Source: CAD feature listing. Evaluate the final solid. Frame: model axes, mm. Face numbers are marked on the shaded views. A direction names the side the tool comes from. Round coordinates to 2 decimals unless told otherwise and drop trailing zeros. Loops run counter-clockwise (first coordinate to the right, second up) from the corner with the lowest first, then second, coordinate; pieces in that order, holes last. Notation, with made-up numbers: M 78.5,13.5 L 126.5,13.5 A20 cw 126.5,42.5 Z; hole C 72,73.25 d5. An arc over 180 degrees is marked long. Write each question's results on one line, items separated by ' | '. Start each with the question number.
1. Set-up query: the marked faces 4, 5 and 6. Return all of +Z, -Z, +X, -X, +Y, -Y with unobstructed straight access to the full face (end or side cutting, diameter ignored); none if empty.
2. Section A-A on x = 2. Output: boundary loops of the cut face in (y, z).
3. Contact query for flat-ended pins moving along their axis: pin 1 Ø10 at (x, z) = (-55, 33) entering from -Y; pin 2 Ø10 at (x, y) = (12.5, -90) entering from -Z; pin 3 Ø10 at (y, z) = (-94, 7.5) entering from +X; pin 4 Ø1.5 at (y, z) = (-40.5, 17.5) entering from -X. Output: stop coordinate, or through.
4. Draft query along Y for the marked faces 1, 2 and 3. Return one class per face: released by +Y, released by -Y, zero draft, split by the parting line, or undercut.
5. Ray query, line 1 (Z direction, x = -22, y = -14.5); line 2 (X direction, y = -14.5, z = 88.5); line 3 (Y direction, x = -10.5, z = 7.5). Return the intervals inside material, ascending.
6. Section D-D on z = 46. Output: boundary loops of the cut face in (x, y), and give its area (3 significant figures).
7. Section B-B on z = 131.5. Output: boundary loops of the cut face in (x, y), and give its area (3 significant figures).
8. Section C-C on y = -50.8. Output: boundary loops of the cut face in (x, z).
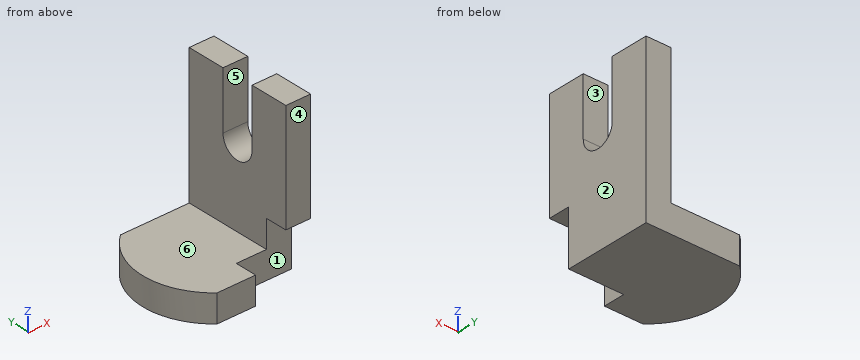
from build123d import *

# Parameters (mm, degrees)
F1_DEPTH = 101.6
F3_DEPTH = 25.401
F4_W     = 50.8
F4_H     = 50.8
F5_DEPTH = 20.32
F7_DEPTH = 22.861


with BuildPart() as f1:
    # F0 (on Front) → F1 (new body)
    with BuildSketch(Plane.XZ):
        Polygon((22.86, 152.4), (0, 152.4), (0, 25.4), (-88.9, 25.4), (-88.9, 0), (0, 0), (22.86, 0), align=None)
    extrude(amount=F1_DEPTH)

    # F2 (on face) → F3 (cut, through all)
    with BuildSketch(Plane.XY.offset(25.4)):
        with BuildLine():
            Line((-88.9, -101.6), (-63.5, -101.6))
            ThreePointArc((-63.5, -101.6), (-87.342351, -50.8), (-63.5, 0))
            Line((-63.5, 0), (-88.9, 0))
            Line((-88.9, 0), (-88.9, -101.6))
        make_face()
    extrude(amount=-F3_DEPTH, mode=Mode.SUBTRACT)

    # F4 (on face) → F5 (cut)
    with BuildSketch(Plane.XZ.offset(101.6)):
        with Locations((-2.54, 25.4)):
            Rectangle(F4_W, F4_H)
    extrude(amount=-F5_DEPTH, mode=Mode.SUBTRACT)

    # F6 (on face) → F7 (cut, through all)
    with BuildSketch(Plane(origin=(0, 0, 0), x_dir=(0, -1, 0), z_dir=(-1, 0, 0))):
        with BuildLine():
            Line((66.04, 152.4), (35.56, 152.4))
            Line((35.56, 152.4), (35.56, 99.06))
            ThreePointArc((35.56, 99.06), (50.8, 83.82), (66.04, 99.06))
            Line((66.04, 99.06), (66.04, 152.4))
        make_face()
    extrude(amount=-F7_DEPTH, mode=Mode.SUBTRACT)


solid = f1.part
Taken from the geometry:
1) face 4: +Z, -Z, +X, -X, -Y | face 5: +Z, +X, -X | face 6: +Z, -X, +Y, -Y
2) outline: M -101.6,50.8 L -81.28,50.8 L -81.28,0 L 0,0 L 0,152.4 L -35.56,152.4 L -35.56,99.06 A15.24 cw -66.04,99.06 L -66.04,152.4 L -101.6,152.4 Z
3) pin 1: through | pin 2: z = 50.8 | pin 3: x = -27.94 | pin 4: x = -86.65
4) face 1: released by -Y | face 2: zero draft | face 3: undercut
5) line 1: 0 to 25.4 | line 2: 0 to 22.86 | line 3: -81.28 to 0
6) outline: M 0,-81.28 L 22.86,-81.28 L 22.86,0 L 0,0 Z | area: 1,860 mm^2
7) outline: M 0,-101.6 L 22.86,-101.6 L 22.86,-66.04 L 0,-66.04 Z; M 0,-35.56 L 22.86,-35.56 L 22.86,0 L 0,0 Z | area: 1,630 mm^2
8) outline: M -87.34,0 L 22.86,0 L 22.86,83.82 L 0,83.82 L 0,25.4 L -87.34,25.4 Z
